from build123d import *

# Parameters (mm, degrees)
SKETCH2_R           = 5.525
BOSS_EXTRUDE1_DEPTH = 10
SKETCH4_R           = 5
BOSS_EXTRUDE3_DEPTH = 7
SKETCH5_R           = 5.525
SKETCH5_R_2         = 4.5
BOSS_EXTRUDE4_DEPTH = 6
BOSS_EXTRUDE5_DEPTH = 15


with BuildPart() as part:
    # Sketch2 → Boss-Extrude1 (new body)
    with BuildSketch(Plane.XY):
        with BuildLine():
            Line((-88.62562975, -17.425503603), (11.37437025, -17.425503603))
            Line((11.37437025, -17.425503603), (11.37437025, 2.574496397))
            Line((11.37437025, 2.574496397), (11.37437025, 66.938471641))
            ThreePointArc((11.37437025, 66.938471641), (2.08841102, 80.807492446), (-14.272261494, 77.504891684))
            Line((-14.272261494, 77.504891684), (-87.174506998, 4.049231386))
            ThreePointArc((-87.174506998, 4.049231386), (-88.248636685, 2.431771629), (-88.62562975, 0.527091372))
            Line((-88.62562975, 0.527091372), (-88.62562975, -17.425503603))
        make_face()
        with Locations((-3.62562975, 66.938471641)):
            Circle(SKETCH2_R, mode=Mode.SUBTRACT)
        with BuildLine():
            Line((-15.629426982, 20.624496397), (-21.07612441, 20.624496397))
            ThreePointArc((-21.07612441, 20.624496397), (-25.154426982, 11.599496397), (-21.07612441, 2.574496397))
            Line((-21.07612441, 2.574496397), (-5.182729555, 2.574496397))
            ThreePointArc((-5.182729555, 2.574496397), (-1.104426982, 11.599496397), (-5.182729555, 20.624496397))
            Line((-5.182729555, 20.624496397), (-10.629426982, 20.624496397))
            Line((-10.629426982, 20.624496397), (-10.629426982, 25.624496397))
            Line((-10.629426982, 25.624496397), (-5.241089336, 25.624496397))
            ThreePointArc((-5.241089336, 25.624496397), (-1.714029472, 27.080508712), (-0.241146646, 30.600556911))
            Line((-0.241146646, 30.600556911), (-0.142030474, 51.301718396))
            ThreePointArc((-0.142030474, 51.301718396), (-1.43979486, 54.662291481), (-4.659411057, 56.278371739))
            ThreePointArc((-4.659411057, 56.278371739), (-7.11800033, 56.813760216), (-9.38382576, 57.907989239))
            ThreePointArc((-9.38382576, 57.907989239), (-12.624755601, 58.661476378), (-15.620909093, 57.214260654))
            Line((-15.620909093, 57.214260654), (-60.051592087, 12.446295905))
            ThreePointArc((-60.051592087, 12.446295905), (-61.255836785, 6.063207717), (-55.776519908, 2.574496397))
            Line((-55.776519908, 2.574496397), (-27.565492929, 2.574496397))
            ThreePointArc((-27.565492929, 2.574496397), (-29.975609484, 14.060544979), (-24.380364504, 24.37709515))
            ThreePointArc((-24.380364504, 24.37709515), (-22.842052811, 25.302262625), (-21.07612441, 25.624496397))
            Line((-21.07612441, 25.624496397), (-15.629426982, 25.624496397))
            Line((-15.629426982, 25.624496397), (-15.629426982, 20.624496397))
        make_face(mode=Mode.SUBTRACT)
    extrude(amount=BOSS_EXTRUDE1_DEPTH)

    # Sketch4 → Boss-Extrude3 (add)
    with BuildSketch(Plane.XZ.offset(17.425503603)):
        with BuildLine():
            ThreePointArc((6.37437025, 12.5), (0.080275025, 17.329629131), (-2.955756769, 10))
            Line((-2.955756769, 10), (5.704497269, 10))
            ThreePointArc((5.704497269, 10), (6.203999382, 11.205904774), (6.37437025, 12.5))
        make_face()
        with BuildLine():
            Line((5.704497269, 10), (-2.955756769, 10))
            ThreePointArc((-2.955756769, 10), (-1.125629745, 8.169872978), (1.374370261, 7.5))
            ThreePointArc((1.374370261, 7.5), (3.874370255, 8.169872984), (5.704497269, 10))
        make_face()
        with Locations((-78.62562975, 12.5)):
            Circle(SKETCH4_R)
    extrude(amount=-BOSS_EXTRUDE3_DEPTH)

    # Sketch5 → Boss-Extrude4 (add)
    with BuildSketch(Plane(origin=(0, 0, 0), x_dir=(-1, 0, 0), z_dir=(0, 0, -1))):
        with Locations((3.62562975, 66.938471641)):
            Circle(SKETCH5_R)
        with Locations((3.62562975, 66.938471641)):
            Circle(SKETCH5_R_2, mode=Mode.SUBTRACT)
    extrude(amount=-BOSS_EXTRUDE4_DEPTH)

    # Sketch6 → Boss-Extrude5 (add)
    with BuildSketch(Plane.XY.offset(10)):
        with BuildLine():
            Line((-24.542139193, 2.574496397), (-1.716714772, 2.574496397))
            ThreePointArc((-1.716714772, 2.574496397), (-0.342785676, 1.676425663), (-0.614037264, 0.057588185))
            ThreePointArc((-0.614037264, 0.057588185), (-13.129426982, -5.425503603), (-25.644816701, 0.057588185))
            ThreePointArc((-25.644816701, 0.057588185), (-25.916068288, 1.676425663), (-24.542139193, 2.574496397))
        make_face()
    extrude(amount=BOSS_EXTRUDE5_DEPTH)


solid = part.part
Check sheet for the modelled part. Datum: model origin and axes. Units: mm. A direction names the side the tool comes from. Give positions to 0.01 mm unless a question says otherwise; leave off trailing zeros. Write each loop counter-clockwise with the first axis right and the second up, starting at its lowest first coordinate (ties: lowest second). Pieces come first, ordered by that corner, then holes. Notation, with made-up numbers: M -22,5 L 13,5 A27 ccw 13,31 Z; hole C -13,45 d1. An arc over 180 degrees is marked long. Use one line per item in the form item = value.
(1) Section check D-D on y = -9. Record the boundary of the cut face in (x, z), plus the area to 3 significant figures.
Answer block:
outline = M -88.63,0 L 11.37,0 L 11.37,10 L -88.63,10 Z
area = 1,000 mm2
(2) Section check A-A on z = 3.5. State how many separate pieces and enclosed holes the cut face has, plus the area to 3 significant figures.
Answer block:
separate_pieces = 1
enclosed_holes = 2
area = 4,660 mm2
(3) Draft check along Y on faces 1 (the cylindrical face through (-25.926, 1.654, 17.395)), 2 (the cylindrical face through (-1.105, 11.457, 4.93)), 3 (the cylindrical face through (2.32, 80.71, 4.93)). Enter one of: pulls with the +Y half, pulls with the -Y half, needs draft (parallel to the pull), parting line crosses it, or undercut.
Answer block:
face_1 = parting line crosses it
face_2 = undercut
face_3 = pulls with the +Y half
(4) Section check B-B on x = -42.5. Record the boundary of the cut face in (y, z), plus the area to 3 significant figures.
Answer block:
outline = M -17.43,0 L 2.57,0 L 2.57,10 L -17.43,10 Z; M 30.13,0 L 49.06,0 L 49.06,10 L 30.13,10 Z
area = 389 mm2
(5) Depth check by flat-ended pin: P1, Ø1.5, axis at x = -43.5, y = -0.5, coming from the +Z side; P2, Ø1.5, axis at y = 22.5, z = 4, coming from the -X side; P3, Ø3.5, axis at x = 1, z = 14, coming from the +Y side. Enter the tip coordinate at first touch or a pass-through.
Answer block:
P1 = 10
P2 = -69.61
P3 = 2.22
(6) Material ranges on line 1 along Y through (x, z) = (-10.5, 1.75); line 2 along X through (y, z) = (11, 7.5); line 3 along Y through (x, z) = (-33, 5.5), recorded low to high.
Answer block:
line_1 = -17.43 to 2.57, 20.62 to 25.62, 58.44 to 80.27
line_2 = -80.28 to -61.1, -30.14 to -25.14, -1.12 to 11.37
line_3 = -17.43 to 2.57, 39.7 to 58.63
(7) Tool access check on faces 4 (the flat face through (1, -10.426, 13)), 5 (the flat face through (-79, -10.426, 13)), 6 (the flat face through (-15.629, 23, 5)). Record the directions out of +Z, -Z, +X, -X, +Y, -Y that give a thin tool (end or side, any length) a straight path to the whole face; none if there is none.
Answer block:
face_4 = +Z, +X, -X
face_5 = +Z, +X, -X, +Y
face_6 = +Z, -Z
(8) Section check C-C on y = 70. Record the boundary of the cut face in (x, z), plus the area to 3 significant figures.
Answer block:
outline = M -21.72,0 L -6.92,0 L -6.92,6 L -8.22,6 L -8.22,10 L -21.72,10 Z; M -0.33,0 L 11.06,0 L 11.06,10 L 0.97,10 L 0.97,6 L -0.33,6 Z
area = 251 mm2
